from build123d import *

# Parameters (mm, degrees)
BOSS_EXTRUDE1_DEPTH              = 15.24
TAP_DRILL_FOR_M10X1_0_TAP1_D     = 7.62
TAP_DRILL_FOR_M10X1_0_TAP1_DEPTH = 7.62
TAP_DRILL_FOR_M10X1_0_TAP1_TIP   = 2.289278958
TAP_DRILL_FOR_M10X1_0_TAP3_D     = 6.35
TAP_DRILL_FOR_M10X1_0_TAP3_DEPTH = 7.62
TAP_DRILL_FOR_M10X1_0_TAP3_TIP   = 1.907732465


with BuildPart() as part:
    # Sketch1 → Boss-Extrude1 (new body)
    with BuildSketch(Plane(origin=(0, 0, 0), x_dir=(1, 0, 0), z_dir=(0, 1, 0))):
        with BuildLine():
            Line((-39.37, 0), (-55.240527947, 0))
            Line((-55.240527947, 0), (-55.240527947, -7.62))
            Line((-55.240527947, -7.62), (-45.080527947, -7.62))
            ThreePointArc((-45.080527947, -7.62), (-33.007335275, -31.635963998), (-9.525, -44.716806404))
            Line((-9.525, -44.716806404), (-9.525, -76.2))
            Line((-9.525, -76.2), (9.525, -76.2))
            Line((9.525, -76.2), (9.525, -44.716806404))
            ThreePointArc((9.525, -44.716806404), (33.007335275, -31.635963998), (45.080527947, -7.62))
            Line((45.080527947, -7.62), (55.240527947, -7.62))
            Line((55.240527947, -7.62), (55.240527947, 0))
            Line((55.240527947, 0), (39.37, 0))
            ThreePointArc((39.37, 0), (0, -39.37), (-39.37, 0))
        make_face()
    extrude(amount=BOSS_EXTRUDE1_DEPTH)

    # Tap Drill for M10x1.0 Tap1
    with Locations(Plane.XY.offset(76.2)):
        with Locations((0, 7.62)):
            Hole(TAP_DRILL_FOR_M10X1_0_TAP1_D / 2, depth=TAP_DRILL_FOR_M10X1_0_TAP1_DEPTH)
            with Locations((0, 0, -(TAP_DRILL_FOR_M10X1_0_TAP1_DEPTH + TAP_DRILL_FOR_M10X1_0_TAP1_TIP / 2))):  # 118° drill point
                Cone(0, TAP_DRILL_FOR_M10X1_0_TAP1_D / 2, TAP_DRILL_FOR_M10X1_0_TAP1_TIP, mode=Mode.SUBTRACT)

    # Tap Drill for M10x1.0 Tap3
    with Locations(Plane.XY.offset(7.62)):
        with Locations((-50.160527947, 7.62), (50.160527947, 7.62)):
            Hole(TAP_DRILL_FOR_M10X1_0_TAP3_D / 2, depth=TAP_DRILL_FOR_M10X1_0_TAP3_DEPTH)
            with Locations((0, 0, -(TAP_DRILL_FOR_M10X1_0_TAP3_DEPTH + TAP_DRILL_FOR_M10X1_0_TAP3_TIP / 2))):  # 118° drill point
                Cone(0, TAP_DRILL_FOR_M10X1_0_TAP3_D / 2, TAP_DRILL_FOR_M10X1_0_TAP3_TIP, mode=Mode.SUBTRACT)


solid = part.part
Input: part model. Units: mm. Frame: model coordinates. A direction names the side the tool comes from. Coordinates: 2 decimals unless noted, no trailing zeros. Loops run counter-clockwise (first coordinate to the right, second up) from the corner with the lowest first, then second, coordinate; pieces in that order, holes last. Notation, with made-up numbers: (-8, 26.25) -> (33, 26.25) arc R24 cw to (33, 58.25) -> close; hole circle Ø11 at (-25, 47.5). An arc over 180 degrees is marked (long way). Write each question's results on one line, items separated by ' | '. Start each with the question number.
Q1. Section A-A, the plane z = 19. Return the cut outline in (x, y), plus the area to 3 significant figures.
Q2. Section C-C, the plane x = 19.5. Return the cut outline in (y, z).
Q3. Ray query, line 1 (Y direction, x = 0, z = 73.75); line 2 (X direction, y = 7.62, z = 2.75); line 3 (X direction, y = 4.75, z = 63) (3 decimals). Return the intervals inside material, ascending. Write a range as from..to.
Q4. Section D-D, the plane y = 6.5. State how many separate pieces and enclosed holes the cut face has, plus the area to 3 significant figures.
Q5. Reachability of faces 1 (the flat face through (-9.525, 8, 60)), 2 (the cylindrical face through (0.496, 11.398, 72.337)), 3 (the flat face through (9.525, 8, 61)) from +Z, -Z, +X, -X, +Y, -Y: full face, straight path, thin tool, end or side. Return the list, or none.
Q6. Section B-B, the plane y = 1.25. Return the cut outline in (x, z) (3 decimals).
Q7. Pin query (flat end, axial travel): pin 1 (5 mm diameter, centred on x = -50.16, y = 7.62, fed in from -Z); pin 2 (6 mm diameter, centred on x = -26.5, y = 13.5, fed in from -Z); pin 3 (8 mm diameter, centred on x = 51, y = 8, fed in from +Z); pin 4 (1.5 mm diameter, centred on y = 6, z = 47.5, fed in from -X) (3 decimals). Return the tip coordinate at first contact, or that it passes through.
Q8. Pull-direction query (Y, two-part tool) for faces 4 (the flat face through (55.241, 8, 4)), 5 (the flat face through (4, 15.24, 41)), 6 (the cylindrical face through (47.23, 6.4, 3.76)); classes: released by +Y, released by -Y, zero draft, split by the parting line, or undercut.
Found:
1) outline: (-41.59, 0) -> (-34.48, 0) -> (-34.48, 15.24) -> (-41.59, 15.24) -> close; (34.48, 0) -> (41.59, 0) -> (41.59, 15.24) -> (34.48, 15.24) -> close | area: 217 mm2
2) outline: (0, 34.2) -> (15.24, 34.2) -> (15.24, 41.35) -> (0, 41.35) -> close
3) line 1: 0..3.81, 11.43..15.24 | line 2: -55.24..-53.34, -46.99..-39.27, 39.27..46.99, 53.34..55.24 | line 3: -9.525..9.525
4) separate pieces: 3 | enclosed holes: 0 | area: 1,430 mm2
5) face 1: +Z, -X, +Y, -Y | face 2: +Z | face 3: +Z, +X, +Y, -Y
6) outline: (-55.241, 0) -> (-39.37, 0) arc R39.37 cw to (39.37, 0) -> (55.241, 0) -> (55.241, 7.62) -> (45.081, 7.62) arc R45.72 ccw to (9.525, 44.717) -> (9.525, 76.2) -> (-9.525, 76.2) -> (-9.525, 44.717) arc R45.72 ccw to (-45.081, 7.62) -> (-55.241, 7.62) -> close
7) pin 1: through | pin 2: z = 26.07 | pin 3: z = 7.62 | pin 4: x = -9.525
8) face 4: zero draft | face 5: released by +Y | face 6: undercut
